```python
from build123d import *

# Parameters (mm, degrees)
SKETCH1_R               = 18.5
SKETCH1_R_2             = 12.5
BOSS_EXTRUDE1_DEPTH     = 6.5
SKETCH2_R               = 46.70286463
CUT_EXTRUDE1_DEPTH      = 27.958301133
CUT_EXTRUDE2_DEPTH      = 27.958301133
CUT_EXTRUDE2_DEPTH_BACK = 27.958301133
SKETCH3_R               = 1.125
SKETCH4_R               = 1.9
CUT_EXTRUDE3_DEPTH      = 23.989128026
BOSS_EXTRUDE2_START     = 12.5
SKETCH6_W               = 6
SKETCH6_H               = 6.5
SKETCH6_R               = 1.125
BOSS_EXTRUDE2_DEPTH     = 12.5
CUT_EXTRUDE4_START      = -12.5
SKETCH7_R               = 1.9
CUT_EXTRUDE4_DEPTH      = 12.5
BOSS_EXTRUDE3_DEPTH     = 6.5
CUT_EXTRUDE7_DEPTH      = 12.5
FILLET2_R               = 3
SKETCH14_R              = 1
CUT_EXTRUDE9_DEPTH      = 33.805335008
BOSS_EXTRUDE4_START     = 12.5
SKETCH15_W              = 7.3
SKETCH15_H              = 6.5
SKETCH15_R              = 1
BOSS_EXTRUDE4_DEPTH     = 12.5
FILLET3_R               = 10
SKETCH16_R              = 1.9
CUT_EXTRUDE11_DEPTH     = 37.526565832


with BuildPart() as part:
    # Sketch1 → Boss-Extrude1 (new body)
    with BuildSketch(Plane(origin=(0, 0, 0), x_dir=(1, 0, 0), z_dir=(0, 1, 0))):
        with Locations(Location((0, 0, 0), (0, 0, 90))):
            Circle(SKETCH1_R)
        with Locations(Location((0, 0, 0), (0, 0, 90))):
            Circle(SKETCH1_R_2, mode=Mode.SUBTRACT)
    extrude(amount=BOSS_EXTRUDE1_DEPTH)

    # Sketch2 → Cut-Extrude1 (cut, through all)
    with BuildSketch(Plane(origin=(0, 0, 0), x_dir=(0, 0, -1), z_dir=(1, 0, 0))):
        Circle(SKETCH2_R)
    extrude(amount=CUT_EXTRUDE1_DEPTH, mode=Mode.SUBTRACT)

    # Sketch3 → Cut-Extrude2 (cut, two sides: drawn at the far end of the back side and taken through both)
    with BuildSketch(Plane(origin=(0, 0, 0), x_dir=(0, 0, -1), z_dir=(1, 0, 0)).offset(-CUT_EXTRUDE2_DEPTH_BACK)):
        with Locations((14.7, 3.25)):
            Circle(SKETCH3_R)
    extrude(amount=CUT_EXTRUDE2_DEPTH + CUT_EXTRUDE2_DEPTH_BACK, mode=Mode.SUBTRACT)

    # Sketch4 → Cut-Extrude3 (cut, through all)
    with BuildSketch(Plane(origin=(-6.5, 0, 0), x_dir=(0, 0, -1), z_dir=(1, 0, 0))):
        with Locations((14.7, 3.25)):
            Circle(SKETCH4_R)
    extrude(amount=-CUT_EXTRUDE3_DEPTH, mode=Mode.SUBTRACT)

    # Sketch6 → Boss-Extrude2 (add)
    with BuildSketch(Plane(origin=(0, 0, 0), x_dir=(0, 0, -1), z_dir=(1, 0, 0)).offset(BOSS_EXTRUDE2_START)):
        with Locations((15.5, 3.25)):
            Rectangle(SKETCH6_W, SKETCH6_H)
        with Locations((14.7, 3.25)):
            Circle(SKETCH6_R, mode=Mode.SUBTRACT)
    extrude(amount=-BOSS_EXTRUDE2_DEPTH)

    # Sketch7 → Cut-Extrude4 (cut)
    with BuildSketch(Plane.ZY.offset(6.5).offset(CUT_EXTRUDE4_START)):
        with Locations(Location((-14.7, 3.25, 0), (0, 0, 180))):
            Circle(SKETCH7_R)
    extrude(amount=CUT_EXTRUDE4_DEPTH, mode=Mode.SUBTRACT)

    # Sketch11 → Boss-Extrude3 (add)
    with BuildSketch(Plane(origin=(0, 0, 0), x_dir=(1, 0, 0), z_dir=(0, 1, 0))):
        with BuildLine():
            Line((0, -18.5), (0, -26.3))
            ThreePointArc((0, -26.3), (-13.323632383, -16.015482855), (-18.5, 0))
            ThreePointArc((-18.5, 0), (-13.015505379, -13.015505379), (0, -18.5))
        make_face()
    extrude(amount=BOSS_EXTRUDE3_DEPTH)

    # Sketch13 → Cut-Extrude7 (cut)
    with BuildSketch(Plane(origin=(0, 0, 0), x_dir=(-1, 0, 0), z_dir=(0, -1, 0))):
        with BuildLine():
            ThreePointArc((8.831682782, -8.845980965), (4.778872144, -11.550427742), (0, -12.5))
            Line((0, -12.5), (0, -19))
            ThreePointArc((0, -19), (5.098309427, -15.844292422), (9.082430599, -11.363441184))
            Line((9.082430599, -11.363441184), (8.831682782, -8.845980965))
        make_face()
    extrude(amount=-CUT_EXTRUDE7_DEPTH, mode=Mode.SUBTRACT)

    # Fillet2
    fillet2_edges = [part.edges().sort_by_distance(p)[0] for p in [
        (-8.831682782, 3.25, 8.845980965),
    ]]
    fillet(fillet2_edges, radius=FILLET2_R)

    # Sketch14 → Cut-Extrude9 (cut, through all)
    with BuildSketch(Plane(origin=(0, 0, 0), x_dir=(0, 0, -1), z_dir=(1, 0, 0))):
        with Locations((-22.5, 3.25)):
            Circle(SKETCH14_R)
    extrude(amount=-CUT_EXTRUDE9_DEPTH, mode=Mode.SUBTRACT)

    # Sketch15 → Boss-Extrude4 (add)
    with BuildSketch(Plane(origin=(0, 0, 0), x_dir=(0, 0, -1), z_dir=(1, 0, 0)).offset(BOSS_EXTRUDE4_START)):
        with Locations((-22.65, 3.25)):
            Rectangle(SKETCH15_W, SKETCH15_H)
        with Locations((-22.5, 3.25)):
            Circle(SKETCH15_R, mode=Mode.SUBTRACT)
    extrude(amount=-BOSS_EXTRUDE4_DEPTH)

    # Fillet3
    fillet3_edges = [part.edges().sort_by_distance(p)[0] for p in [
        (0, 3.25, 19),
    ]]
    fillet(fillet3_edges, radius=FILLET3_R)

    # Sketch16 → Cut-Extrude11 (cut, through all)
    with BuildSketch(Plane(origin=(6, 0, 0), x_dir=(0, 0, -1), z_dir=(1, 0, 0))):
        with Locations((-22.5, 3.25)):
            Circle(SKETCH16_R)
    extrude(amount=-CUT_EXTRUDE11_DEPTH, mode=Mode.SUBTRACT)


solid = part.part
```
Build history of the part. All positions in model axes, mm. A direction names the side the tool comes from. Round coordinates to 2 decimals unless told otherwise and drop trailing zeros. Order: outer loops, then holes, each group sorted by start corner. A loop starts at its lowest first (then second) coordinate and runs counter-clockwise, first axis right, second up. Notation, with made-up numbers: (66.25, 40) -> (79.25, 40) arc R18 ccw to (79.25, 53) -> close; hole circle Ø11 at (-28, -1). An arc over 180 degrees is marked (long way). Answer in a Markdown table with one row per item.
1) Band-saw the part on B-B on y = 3.25. Give the number of separate pieces and of enclosed holes in the cut face, and give its area (3 significant figures).
Values:
| item | result |
|---|---|
| separate pieces | 3 |
| enclosed holes | 0 |
| area | 359 mm2 |
2) Band-saw the part on C-C on z = -14.7. Give the cut face in (x, y) (3 decimals), and give its area (3 significant figures).
Values:
| item | result |
|---|---|
| outline | (-11.232, 0) -> (12.5, 0) -> (12.5, 2.125) -> (6, 2.125) -> (6, 1.35) -> (-11.232, 1.35) -> close; (-11.232, 5.15) -> (6, 5.15) -> (6, 4.375) -> (12.5, 4.375) -> (12.5, 6.5) -> (-11.232, 6.5) -> close |
| area | 74.2 mm2 |
3) Which spindle directions (+Z, -Z, +X, -X, +Y, -Y) get a long thin tool onto all of the face, cutting with end or side? Do faces 4 (the flat face through (-10, 0, 9)), 5 (the cylindrical face through (-1.4, 3.3, -12.8)), 6 (the cylindrical face through (-0.43, 3.3, 18.58)). Say none if no direction does.
Values:
| item | result |
|---|---|
| face 4 | +Z, -Z, +X, -X, -Y |
| face 5 | -X |
| face 6 | +X, +Y, -Y |
4) Mould opens along Y. For faces 1 (the flat face through (-9.024, 3.204, 10.775)), 2 (the flat face through (-10, 6.5, 9)), 3 (the cylindrical face through (0.158, 3.821, 20.688)) say: released by +Y, released by -Y, zero draft, split by the parting line, or undercut.
Values:
| item | result |
|---|---|
| face 1 | zero draft |
| face 2 | released by +Y |
| face 3 | undercut |
5) Band-saw the part on A-A on x = 3. Give the cut face in (y, z), and give its area (3 significant figures).
Values:
| item | result |
|---|---|
| outline | (0, -18.5) -> (6.5, -18.5) -> (6.5, -12.5) -> (0, -12.5) -> close; (0, 19) -> (6.5, 19) -> (6.5, 26.3) -> (0, 26.3) -> close; hole circle Ø3.8 at (3.25, -14.7); hole circle Ø3.8 at (3.25, 22.5) |
| area | 63.8 mm2 |
6) Band-saw the part on D-D on x = 8. Give the cut face in (y, z) (3 decimals), and give its area (3 significant figures).
Values:
| item | result |
|---|---|
| outline | (0, -18.5) -> (6.5, -18.5) -> (6.5, -12.5) -> (0, -12.5) -> close; (0, 19) -> (6.5, 19) -> (6.5, 26.3) -> (0, 26.3) -> close; hole circle Ø2.25 at (3.25, -14.7); hole circle Ø2 at (3.25, 22.5) |
| area | 79.3 mm2 |
7) Pin check, flat tips, straight feed: P1, Ø1.5, axis at y = 3.5, z = -3.5, coming from the +X side; P2, Ø2, axis at x = -8, y = 5, coming from the +Z side; P3, Ø1.5, axis at y = 3.5, z = 19.5, coming from the -X side. Stop position of each tip, or through.
Values:
| item | result |
|---|---|
| P1 | x = -11.76 |
| P2 | z = 22.49 |
| P3 | x = -11.14 |
8) Wall check: L1, parallel to Y at x = -4.25, z = 22.5; L2, parallel to Z at x = 11.5, y = 6; L3, parallel to Z at x = -4, y = 4.5. Give the ranges that are in metal, low to high.
Values:
| item | result |
|---|---|
| L1 | 0 to 1.35, 5.15 to 6.5 |
| L2 | -18.5 to -12.5, 19 to 26.3 |
| L3 | -18.06 to -16.13, -13.27 to -11.84, 16.71 to 21.07, 23.93 to 24.44 |
